Check sheet for the modelled part. Datum: model origin and axes. Units: mm. Face numbers are marked on the shaded views. A direction names the side the tool comes from. Give positions to 0.01 mm unless a question says otherwise; leave off trailing zeros. Order: outer loops, then holes, each group sorted by start corner. A loop starts at its lowest first (then second) coordinate and runs counter-clockwise, first axis right, second up. Notation, with made-up numbers: (83.25, 37.25) - (87.25, 37.25) arc R17 cw to (87.25, 51.25) - close; hole circle Ø4 at (10.25, 43.5). An arc over 180 degrees is marked (long way). Answer in a Markdown table with one row per item.
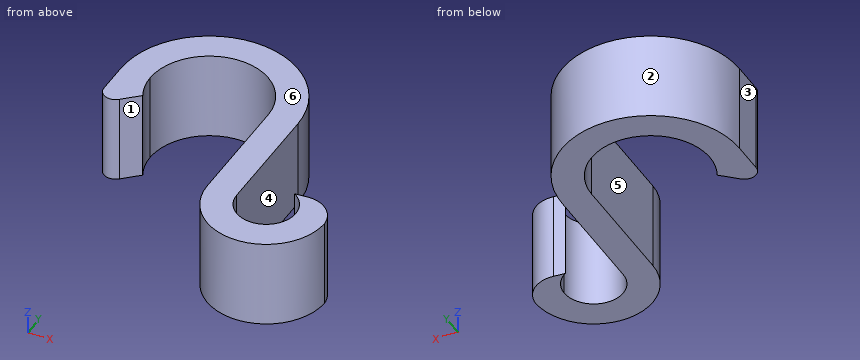
from build123d import *

# Parameters (mm, degrees)
F0_W     = 6.35
F0_H     = 25.4
F1_DEPTH = 19.05
F2_R     = 2.54


with BuildPart() as f1:
    # F0 (on Top) → F1 (new body)
    with BuildSketch(Plane.XY):
        with BuildLine():
            ThreePointArc((-50.8, 9.50515), (-38.1, 22.20515), (-25.4, 9.50515))
            Line((-25.4, 9.50515), (-19.05, 9.50515))
            ThreePointArc((-19.05, 9.50515), (-38.1, 28.55515), (-57.15, 9.50515))
            Line((-57.15, 9.50515), (-57.15, -3.19485))
            Line((-57.15, -3.19485), (-49.473359, 3.853894))
            ThreePointArc((-49.473359, 3.853894), (-50.463892, 6.602709), (-50.8, 9.50515))
        make_face()
        with Locations((-22.225, -3.19485)):
            Rectangle(F0_W, F0_H)
        with BuildLine():
            Line((-19.05, -15.89485), (-25.4, -15.89485))
            ThreePointArc((-25.4, -15.89485), (-12.88999, -28.593429), (-0.005684, -16.274787))
            ThreePointArc((-0.005684, -16.274787), (-2.183514, -11.751451), (-6.965598, -10.223322))
            Line((-6.965598, -10.223322), (-9.413118, -10.461719))
            ThreePointArc((-9.413118, -10.461719), (-7.168536, -12.776292), (-6.35, -15.89485))
            ThreePointArc((-6.35, -15.89485), (-12.7, -22.24485), (-19.05, -15.89485))
        make_face()
    extrude(amount=F1_DEPTH)

    # F2
    f2_edges = [f1.edges().sort_by_distance(p)[0] for p in [
        (-57.15, -3.19485, 9.525),
    ]]
    fillet(f2_edges, radius=F2_R)


solid = f1.part
(1) Cross-section at D-D, the plane y = -8. Record the cut outline in (x, z), then the cut area to 3 significant figures.
Geometry says:
| item | result |
|---|---|
| outline | (-25.4, 0) - (-19.05, 0) - (-19.05, 19.05) - (-25.4, 19.05) - close |
| area | 121 mm² |
(2) Cross-section at A-A, the plane y = 5. Record the cut outline in (x, z), then the cut area to 3 significant figures.
Geometry says:
| item | result |
|---|---|
| outline | (-57.15, 0) - (-49.97, 0) - (-49.97, 19.05) - (-57.15, 19.05) - close; (-25.4, 0) - (-19.05, 0) - (-19.05, 19.05) - (-25.4, 19.05) - close |
| area | 258 mm² |
(3) Cross-section at C-C, the plane x = -8. Record the cut outline in (y, z).
Geometry says:
| item | result |
|---|---|
| outline | (-27.69, 0) - (-20.16, 0) - (-20.16, 19.05) - (-27.69, 19.05) - close; (-11.62, 0) - (-10.32, 0) - (-10.32, 19.05) - (-11.62, 19.05) - close |
(4) Gauge pin test, flat ends, axial feed: P1, Ø1.5, axis at x = -27.5, z = 13.5, coming from the -Y side; P2, Ø2, axis at x = -31.5, z = 4, coming from the -Y side; P3, Ø5.5, axis at y = 3, z = 9.5, coming from the +X side. Record the tip position at first contact, or that the pin passes through.
Geometry says:
| item | result |
|---|---|
| P1 | y = 15.2 |
| P2 | y = 19.68 |
| P3 | x = -19.05 |
(5) Thickness scan on L1, parallel to X at y = 9, z = 3.25; L2, parallel to X at y = -4, z = 10.5; L3, parallel to X at y = 20.5, z = 3. Record the ranges inside material, lowest first.
Geometry says:
| item | result |
|---|---|
| L1 | -57.15 to -50.79, -25.4 to -19.05 |
| L2 | -25.4 to -19.05 |
| L3 | -53.66 to -44.46, -31.74 to -22.54 |
(6) Access from +Z, -Z, +X, -X, +Y, -Y to the whole of each face (thin tool, end or side, straight path). Record for the marked faces 4, 5 and 6.
Geometry says:
| item | result |
|---|---|
| face 4 | +Z, -Z, +Y |
| face 5 | +Z, -Z, -Y |
| face 6 | +Z, +X, -X, +Y, -Y |
(7) Mould release check, pull along X, two halves, no side actions. Record for the marked faces 1, 2 and 3: pulls with the +X half, pulls with the -X half, needs draft (parallel to the pull), parting line crosses it, or undercut.
Geometry says:
| item | result |
|---|---|
| face 1 | undercut |
| face 2 | parting line crosses it |
| face 3 | pulls with the -X half |
(8) Cross-section at B-B, the plane z = 1. Record the cut outline in (x, y), then the cut area to 3 significant figures.
Geometry says:
| item | result |
|---|---|
| outline | (-57.15, 2.59) arc R2.54 ccw to (-52.89, 0.71) - (-49.47, 3.85) arc R12.7 cw to (-50.8, 9.51) arc R12.7 cw to (-25.4, 9.51) - (-25.4, -15.89) arc R12.7 ccw to (-0.01, -16.27) arc R6.35 ccw to (-6.97, -10.22) - (-9.41, -10.46) arc R6.35 cw to (-6.35, -15.89) arc R6.35 cw to (-19.05, -15.89) - (-19.05, 9.51) arc R19.05 ccw to (-57.15, 9.51) - close |
| area | 759 mm² |
